Can you work these out from the model? Positions are in its coordinate system, mm. Face numbers are marked on the shaded views. A direction names the side the tool comes from. Round coordinates to 2 decimals unless told otherwise and drop trailing zeros. Write each loop counter-clockwise with the first axis right and the second up, starting at its lowest first coordinate (ties: lowest second). Pieces come first, ordered by that corner, then holes. Notation, with made-up numbers: (-6.5, 10.25) -> (-0.5, 10.25) arc R10 ccw to (-0.5, 16.25) -> close; hole circle Ø11 at (60.25, -37). An arc over 180 degrees is marked (long way). Write item = value, one per line. Start each with the question number.
1) Imagine slicing it at C-C, the plane z = 54. Please give me the cut outline in (x, y).
2) Thinking about a two-plate mould opening in X: for the marked faces 3, 4 and 5, which applies, +X half, -X half, draft (parallel to the pull), parting line (faces both ways), or undercut?
3) Imagine slicing it at A-A, the plane x = 472.5. Please give me the cut outline in (y, z), then the cut area to 3 significant figures.
4) For the marked faces 1 and 2, which set-ups out of +Z, -Z, +X, -X, +Y, -Y let a thin tool reach every point of the face, with its end or its side?
5) If I drill on line 1 (X direction, y = 255, z = 55); line 2 (Y direction, x = 591, z = 54); line 3 (Y direction, x = 487, z = 141.5), over which ranges is the centre line in solid material (lowest first)?
6) Imagine slicing it at B-B, the plane z = 190.5. Please give me the cut outline in (x, y), then the cut area to 3 significant figures.
7) Imagine slicing it at D-D, the plane y = 60. Please give me the cut outline in (x, z), then the cut area to 3 significant figures.
8) I'm going to push a flat-ended pin straight in: pin 1 (3 mm diameter, centred on x = 418, y = 359, fed in from +Z). Where does the tip first touch, or does it pass through?
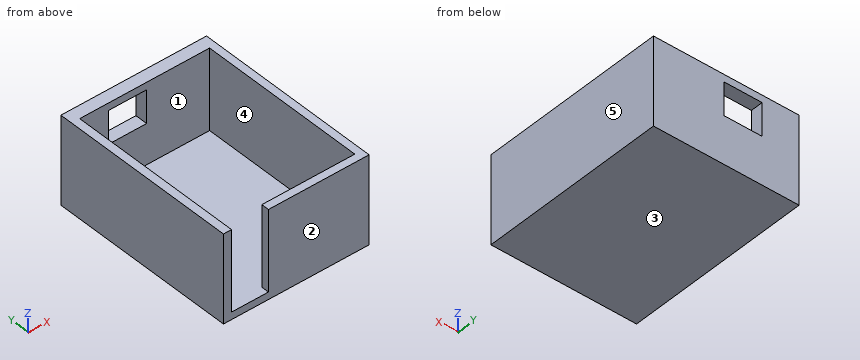
from build123d import *

# Parameters (mm, degrees)
F2_DEPTH = 20
F4_DEPTH = 220
F5_W     = 104
F5_H     = 90
F6_DEPTH = 40


with BuildPart() as f2:
    # F1 (on face) → F2 (new body)
    with BuildSketch(Plane.XY):
        Polygon((413, -75), (688, -75), (688, 440), (290, 440), (290, 406), (290, 141), (290, -75), align=None)
    extrude(amount=F2_DEPTH)

    # F3 (on face) → F4 (join)
    with BuildSketch(Plane.XY.offset(20)):
        Polygon((667, 406), (667, -54), (413, -54), (413, -75), (688, -75), (688, 406), (688, 440), (290, 440), (290, -75), (312, -75), (312, 43), (312, 124), (312, 406), align=None)
    extrude(amount=F4_DEPTH)

    # F5 (on face) → F6 (cut)
    with BuildSketch(Plane(origin=(0, 440, 0), x_dir=(-1, 0, 0), z_dir=(0, 1, 0))):
        with Locations((-443, 175)):
            Rectangle(F5_W, F5_H)
    extrude(amount=-F6_DEPTH, mode=Mode.SUBTRACT)


solid = f2.part
Reported:
q1.outline = (290, -75) -> (312, -75) -> (312, 406) -> (667, 406) -> (667, -54) -> (413, -54) -> (413, -75) -> (688, -75) -> (688, 440) -> (290, 440) -> close
q2.face_3 = draft
q2.face_4 = undercut
q2.face_5 = +X half
q3.outline = (-75, 0) -> (440, 0) -> (440, 130) -> (406, 130) -> (406, 20) -> (-54, 20) -> (-54, 240) -> (-75, 240) -> close; (406, 220) -> (440, 220) -> (440, 240) -> (406, 240) -> close
q3.area = 19,300 mm²
q4.face_1 = +Z
q4.face_2 = +Z, -Z, +X, -X, -Y
q5.line_1 = 290 to 312, 667 to 688
q5.line_2 = -75 to -54, 406 to 440
q5.line_3 = -75 to -54
q6.outline = (290, -75) -> (312, -75) -> (312, 406) -> (391, 406) -> (391, 440) -> (290, 440) -> close; (413, -75) -> (688, -75) -> (688, 440) -> (495, 440) -> (495, 406) -> (667, 406) -> (667, -54) -> (413, -54) -> close
q6.area = 36,000 mm²
q7.outline = (290, 0) -> (688, 0) -> (688, 240) -> (667, 240) -> (667, 20) -> (312, 20) -> (312, 240) -> (290, 240) -> close
q7.area = 17,400 mm²
q8.pin_1 = 20
